```python
from build123d import *

# Parameters (mm, degrees)
SKETCH1_W           = 6
SKETCH1_H           = 19
SKETCH1_H_2         = 6
SKETCH1_W_2         = 19
BOSS_EXTRUDE1_DEPTH = 40
CUT_EXTRUDE1_REACH  = 8
SKETCH2_R           = 10
CUT_EXTRUDE2_REACH  = 27
CUT_EXTRUDE3_DEPTH  = 3
FILLET1_R           = 5


with BuildPart() as part:
    # Sketch1 → Boss-Extrude1 (new body)
    with BuildSketch(Plane(origin=(0, 0, 0), x_dir=(1, 0, 0), z_dir=(0, 1, 0))):
        with Locations((-9.5, 12.5)):
            Rectangle(SKETCH1_W, SKETCH1_H)
        with Locations((-9.5, 0)):
            Rectangle(SKETCH1_W, SKETCH1_H_2)
        with Locations((3, 0)):
            Rectangle(SKETCH1_W_2, SKETCH1_H_2)
    extrude(amount=BOSS_EXTRUDE1_DEPTH)

    # Sketch2 → Cut-Extrude1 (cut, up to next)
    with BuildSketch(Plane(origin=(-6.5, 0, 0), x_dir=(0, 0, -1), z_dir=(1, 0, 0)), mode=Mode.PRIVATE) as cut_extrude1_sk1:
        with Locations((22, 20)):
            Circle(SKETCH2_R)
    cut_extrude1_tool1 = extrude(cut_extrude1_sk1.sketch, amount=-CUT_EXTRUDE1_REACH, mode=Mode.PRIVATE) & part.part
    add(cut_extrude1_tool1.solids().sort_by_distance((-6.5, 20, -22))[0], mode=Mode.SUBTRACT)
    # Sketch2 → Cut-Extrude1 (cut, up to next)
    with BuildSketch(Plane(origin=(-6.5, 0, 0), x_dir=(0, 0, -1), z_dir=(1, 0, 0)), mode=Mode.PRIVATE) as cut_extrude1_sk2:
        with BuildLine():
            Line((9, 35), (9, 25))
            ThreePointArc((9, 25), (7.5, 23.5), (6, 25))
            Line((6, 25), (6, 35))
            ThreePointArc((6, 35), (7.5, 36.5), (9, 35))
        make_face()
    cut_extrude1_tool2 = extrude(cut_extrude1_sk2.sketch, amount=-CUT_EXTRUDE1_REACH, mode=Mode.PRIVATE) & part.part
    add(cut_extrude1_tool2.solids().sort_by_distance((-6.5, 30, -7.5))[0], mode=Mode.SUBTRACT)
    # Sketch2 → Cut-Extrude1 (cut, up to next)
    with BuildSketch(Plane(origin=(-6.5, 0, 0), x_dir=(0, 0, -1), z_dir=(1, 0, 0)), mode=Mode.PRIVATE) as cut_extrude1_sk3:
        with BuildLine():
            Line((9, 5), (9, 15))
            ThreePointArc((9, 15), (7.5, 16.5), (6, 15))
            Line((6, 15), (6, 5))
            ThreePointArc((6, 5), (7.5, 3.5), (9, 5))
        make_face()
    cut_extrude1_tool3 = extrude(cut_extrude1_sk3.sketch, amount=-CUT_EXTRUDE1_REACH, mode=Mode.PRIVATE) & part.part
    add(cut_extrude1_tool3.solids().sort_by_distance((-6.5, 10, -7.5))[0], mode=Mode.SUBTRACT)

    # Sketch3 → Cut-Extrude2 (cut, up to next)
    with BuildSketch(Plane(origin=(0, 0, 3), x_dir=(-1, 0, 0), z_dir=(0, 0, -1)), mode=Mode.PRIVATE) as cut_extrude2_sk1:
        with BuildLine():
            Line((-9, 32.42), (3, 32.42))
            ThreePointArc((3, 32.42), (4.5, 30.92), (3, 29.42))
            Line((3, 29.42), (-9, 29.42))
            ThreePointArc((-9, 29.42), (-10.5, 30.92), (-9, 32.42))
        make_face()
    cut_extrude2_tool1 = extrude(cut_extrude2_sk1.sketch, amount=CUT_EXTRUDE2_REACH, mode=Mode.PRIVATE) & part.part
    add(cut_extrude2_tool1.solids().sort_by_distance((3, 30.92, 3))[0], mode=Mode.SUBTRACT)
    # Sketch3 → Cut-Extrude2 (cut, up to next)
    with BuildSketch(Plane(origin=(0, 0, 3), x_dir=(-1, 0, 0), z_dir=(0, 0, -1)), mode=Mode.PRIVATE) as cut_extrude2_sk2:
        with BuildLine():
            Line((-9, 10.58), (3, 10.58))
            ThreePointArc((3, 10.58), (4.5, 9.08), (3, 7.58))
            Line((3, 7.58), (-9, 7.58))
            ThreePointArc((-9, 7.58), (-10.5, 9.08), (-9, 10.58))
        make_face()
    cut_extrude2_tool2 = extrude(cut_extrude2_sk2.sketch, amount=CUT_EXTRUDE2_REACH, mode=Mode.PRIVATE) & part.part
    add(cut_extrude2_tool2.solids().sort_by_distance((3, 9.08, 3))[0], mode=Mode.SUBTRACT)

    # Sketch4 → Cut-Extrude3 (cut)
    with BuildSketch(Plane(origin=(0, 0, -3), x_dir=(-1, 0, 0), z_dir=(0, 0, -1))):
        with BuildLine():
            Line((-9, 6.33), (3, 6.33))
            ThreePointArc((3, 6.33), (5.75, 9.08), (3, 11.83))
            Line((3, 11.83), (-9, 11.83))
            ThreePointArc((-9, 11.83), (-11.75, 9.08), (-9, 6.33))
        make_face()
        with BuildLine():
            Line((-9, 33.67), (3, 33.67))
            ThreePointArc((3, 33.67), (5.75, 30.92), (3, 28.17))
            Line((3, 28.17), (-9, 28.17))
            ThreePointArc((-9, 28.17), (-11.75, 30.92), (-9, 33.67))
        make_face()
    extrude(amount=-CUT_EXTRUDE3_DEPTH, mode=Mode.SUBTRACT)

    # Fillet1
    fillet1_edges = [part.edges().sort_by_distance(p)[0] for p in [
        (-12.5, 20, 3),
        (12.5, 40, 0),
        (-9.5, 40, -22),
        (-9.5, 30, -22),
        (-9.5, 10, -22),
        (-9.5, 0, -22),
        (12.5, 0, 0),
    ]]
    fillet(fillet1_edges, radius=FILLET1_R)


solid = part.part
```
CAD build for the part. Positions are in the model's coordinates, mm. A direction names the side the tool comes from. Round coordinates to 2 decimals unless told otherwise and drop trailing zeros. Order: outer loops, then holes, each group sorted by start corner. A loop starts at its lowest first (then second) coordinate and runs counter-clockwise, first axis right, second up. Notation, with made-up numbers: (5, -38.5) - (28, -38.5) arc R19 cw to (28, -1.5) - close; hole circle Ø11 at (71, 79.5). An arc over 180 degrees is marked (long way). Answer in a Markdown table with one row per item. Add a question column.
(1) Band-saw the part on A-A on y = 14. List the corners of the cut face in (x, z), and give its area (3 significant figures).
(2) Band-saw the part on D-D on y = 9.5. List the corners of the cut face in (x, z), and give its area (3 significant figures).
(3) 3-axis set-ups, long thin cutter, end or side, ignore diameter. For faces 4 (the face through (-6.5, 20, -10)), 5 (the face through (-9, 30, -6)), 6 (the face through (11.75, 30.86, -1.52)), 7 (the face through (-9.458, 31.22, -21.057)), 8 (the face through (-4.5, 9.1, 1.5)): which of +Z, -Z, +X, -X, +Y, -Y reach the whole face in a straight line?
(4) Mould opens along X. For faces 1 (the face through (11, 38.57, -0.04)), 2 (the face through (-9.5, 36.5, -7.5)), 3 (the face through (3, 32.42, 2)) say: +X half, -X half, draft (parallel to the pull), parting line (faces both ways), or undercut.
(5) Probe L1, parallel to X at y = 30, z = -13; L2, parallel to Z at x = -9.25, y = 5.5; L3, parallel to Z at x = 3.75, y = 35.5. List the from-to ranges inside material, lowest first. Write a range as [from, to].
(6) Band-saw the part on C-C on z = -16.5. List the corners of the cut face in (x, y).
(7) Drop flat-ended pins along their axis: pin 1 Ø3 at (x, y) = (-4, 29) entering from -Z; pin 2 Ø4.5 at (x, y) = (3, 9.5) entering from -Z; pin 3 Ø1 at (x, y) = (-7.5, 17) entering from -Z. Give the stop position or say it passes through.
(8) Band-saw the part on B-B on x = 4.5. List the corners of the cut face in (y, z).
Data:
| question | item | result |
|---|---|---|
| 1 | outline | (-12.5, -14) - (-6.5, -14) - (-6.5, -9) - (-12.5, -9) - close; (-12.5, -6) - (-6.5, -6) - (-6.5, -3) - (12.5, -3) - (12.5, 3) - (-7.5, 3) arc R5 ccw to (-12.5, -2) - close |
| 1 | area | 193 mm^2 |
| 2 | outline | (-12.5, -20.43) - (-6.5, -20.43) - (-6.5, -9) - (-12.5, -9) - close; (-12.5, -6) - (-6.5, -6) - (-6.5, -3) - (-5.72, -3) - (-5.72, 0) - (-4.44, 0) - (-4.44, 3) - (-7.5, 3) arc R5 ccw to (-12.5, -2) - close; (10.44, 0) - (11.72, 0) - (11.72, -3) - (12.5, -3) - (12.5, 3) - (10.44, 3) - close |
| 2 | area | 134 mm^2 |
| 3 | face 4 | -Z, +X, +Y, -Y |
| 3 | face 5 | +X, -X |
| 3 | face 6 | -Z |
| 3 | face 7 | -Z, +X, -X |
| 3 | face 8 | +Z, -Z |
| 4 | face 1 | +X half |
| 4 | face 2 | draft |
| 4 | face 3 | undercut |
| 5 | L1 | x = [-12.5, -6.5] |
| 5 | L2 | z = [-22, -9], [-6, 2.68] |
| 5 | L3 | z = [-3, 3] |
| 6 | outline | (-12.5, 0) - (-6.5, 0) - (-6.5, 11.65) - (-12.5, 11.65) - close; (-12.5, 28.35) - (-6.5, 28.35) - (-6.5, 40) - (-12.5, 40) - close |
| 7 | pin 1 | stops at z = -3 |
| 7 | pin 2 | stops at z = 0 |
| 7 | pin 3 | stops at z = -12.63 |
| 8 | outline | (0, -3) - (6.33, -3) - (6.33, 0) - (7.58, 0) - (7.58, 3) - (0, 3) - close; (10.58, 0) - (11.83, 0) - (11.83, -3) - (28.17, -3) - (28.17, 0) - (29.42, 0) - (29.42, 3) - (10.58, 3) - close; (32.42, 0) - (33.67, 0) - (33.67, -3) - (40, -3) - (40, 3) - (32.42, 3) - close |
